Read the model definition and answer for the solid it produces. Units are mm, in the model's axes. Give positions to 0.01 mm unless a question says otherwise; leave off trailing zeros.
```python
from build123d import *

# Parameters (mm, degrees)
SKETCH1_R           = 2
SKETCH1_R_2         = 2.5
SKETCH1_W           = 4
SKETCH1_H           = 7.5
SKETCH1_H_2         = 6
SKETCH1_W_2         = 10
SKETCH1_H_3         = 4
BOSS_EXTRUDE1_DEPTH = 4


with BuildPart() as part:
    # Sketch1 → Boss-Extrude1 (new body)
    with BuildSketch(Plane(origin=(0, 0, 0), x_dir=(1, 0, 0), z_dir=(0, 1, 0))):
        Polygon((-80, -10.54257408), (-80, 9.45742592), (-100, 29.45742592), (-100, 104.45742592), (-80, 124.45742592), (80, 124.45742592), (100, 104.45742592), (100, 29.45742592), (80, 9.45742592), (80, -10.54257408), (100, -30.54257408), (100, -105.54257408), (80, -125.54257408), (-80, -125.54257408), (-100, -105.54257408), (-100, -30.54257408), align=None)
        with Locations(Location((85, 94.45742592, 0), (0, 0, 270))):
            Circle(SKETCH1_R, mode=Mode.SUBTRACT)
        with Locations(Location((85, 46.45742592, 0), (0, 0, 270))):
            Circle(SKETCH1_R, mode=Mode.SUBTRACT)
        with Locations(Location((85, -95.54257408, 0), (0, 0, 90))):
            Circle(SKETCH1_R, mode=Mode.SUBTRACT)
        with Locations(Location((85, -47.54257408, 0), (0, 0, 90))):
            Circle(SKETCH1_R, mode=Mode.SUBTRACT)
        with Locations(Location((-85, 94.45742592, 0), (0, 0, 90))):
            Circle(SKETCH1_R, mode=Mode.SUBTRACT)
        with Locations(Location((-85, 46.45742592, 0), (0, 0, 90))):
            Circle(SKETCH1_R, mode=Mode.SUBTRACT)
        with Locations(Location((-85, -47.54257408, 0), (0, 0, 270))):
            Circle(SKETCH1_R, mode=Mode.SUBTRACT)
        with Locations(Location((-85, -95.54257408, 0), (0, 0, 270))):
            Circle(SKETCH1_R, mode=Mode.SUBTRACT)
        with Locations(Location((60, 114.45742592, 0), (0, 0, 270))):
            Circle(SKETCH1_R_2, mode=Mode.SUBTRACT)
        with Locations(Location((-60, 114.45742592, 0), (0, 0, 90))):
            Circle(SKETCH1_R_2, mode=Mode.SUBTRACT)
        with Locations(Location((-75, -115.54257408, 0), (0, 0, 270))):
            Circle(SKETCH1_R, mode=Mode.SUBTRACT)
        with Locations(Location((-70, -10.54257408, 0), (0, 0, 270))):
            Circle(SKETCH1_R, mode=Mode.SUBTRACT)
        with Locations(Location((75, -115, 0), (0, 0, 270))):
            Circle(SKETCH1_R, mode=Mode.SUBTRACT)
        with Locations(Location((70, -10.54257408, 0), (0, 0, 270))):
            Circle(SKETCH1_R, mode=Mode.SUBTRACT)
        with BuildLine():
            Line((20, -78.04257408), (-20, -78.04257408))
            ThreePointArc((-20, -78.04257408), (-22.5, -75.54257408), (-20, -73.04257408))
            Line((-20, -73.04257408), (20, -73.04257408))
            ThreePointArc((20, -73.04257408), (22.5, -75.54257408), (20, -78.04257408))
        make_face(mode=Mode.SUBTRACT)
        with BuildLine():
            Line((20, 56.95742592), (-20, 56.95742592))
            ThreePointArc((-20, 56.95742592), (-22.5, 54.45742592), (-20, 51.95742592))
            Line((-20, 51.95742592), (20, 51.95742592))
            ThreePointArc((20, 51.95742592), (22.5, 54.45742592), (20, 56.95742592))
        make_face(mode=Mode.SUBTRACT)
        with Locations((95, -41.25)):
            Rectangle(SKETCH1_W, SKETCH1_H, mode=Mode.SUBTRACT)
        with Locations((95, -96.822248533)):
            Rectangle(SKETCH1_W, SKETCH1_H_2, mode=Mode.SUBTRACT)
        with Locations((70, 8)):
            Rectangle(SKETCH1_W_2, SKETCH1_H_3, mode=Mode.SUBTRACT)
        with Locations((95, -56.25)):
            Rectangle(SKETCH1_W, SKETCH1_H, mode=Mode.SUBTRACT)
        with Locations((50, 8)):
            Rectangle(SKETCH1_W_2, SKETCH1_H_3, mode=Mode.SUBTRACT)
        with Locations((95, -84.822248533)):
            Rectangle(SKETCH1_W, SKETCH1_H_2, mode=Mode.SUBTRACT)
        with Locations((-95, -96.822248533)):
            Rectangle(SKETCH1_W, SKETCH1_H_2, mode=Mode.SUBTRACT)
        with Locations((-95, -84.822248533)):
            Rectangle(SKETCH1_W, SKETCH1_H_2, mode=Mode.SUBTRACT)
        with Locations((-95, -56.25)):
            Rectangle(SKETCH1_W, SKETCH1_H, mode=Mode.SUBTRACT)
        with Locations((-95, -41.25)):
            Rectangle(SKETCH1_W, SKETCH1_H, mode=Mode.SUBTRACT)
        with Locations((-50, 8)):
            Rectangle(SKETCH1_W_2, SKETCH1_H_3, mode=Mode.SUBTRACT)
        with Locations((-70, 8)):
            Rectangle(SKETCH1_W_2, SKETCH1_H_3, mode=Mode.SUBTRACT)
    extrude(amount=BOSS_EXTRUDE1_DEPTH)


solid = part.part
```
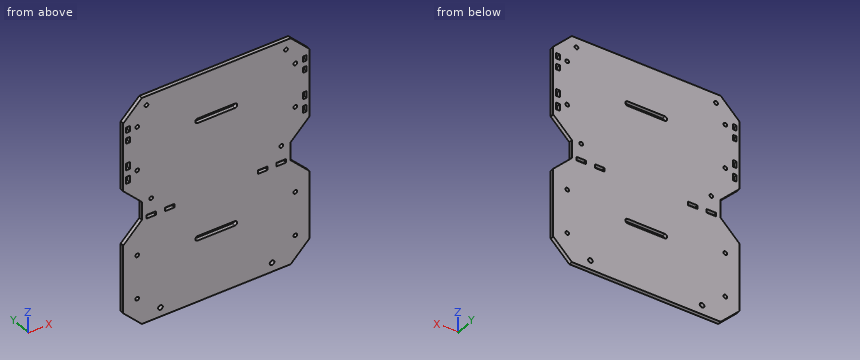
Item 1: Section A-A (y = 1.6) is taken. Give the number of separate pieces and of enclosed holes in the cut face, and give its area (3 significant figures).
Result set:
separate pieces: 1
enclosed holes: 28
area: 46,600 mm2
Item 2: Find the intervals of material crossed by line 1 along Z through (x, y) = (2, 2.85); line 2 along X through (y, z) = (0.6, 57.5); line 3 along Z through (x, y) = (45.5, 2.9), in increasing order.
Result set:
line 1: z = -124.46 to -56.96, -51.96 to 73.04, 78.04 to 125.54
line 2: x = -100 to -97, -93 to 93, 97 to 100
line 3: z = -124.46 to -10, -6 to 125.54
Item 3: Each of these flat-tipped pins is pushed along its axis until it touches: pin 1 Ø4 at (x, z) = (60, -114.46) entering from +Y; pin 2 Ø1.2 at (y, z) = (1.5, -4) entering from -X; pin 3 Ø6 at (x, z) = (-60, -114.46) entering from +Y; pin 4 Ø2 at (x, y) = (94.5, 1) entering from +Z. Where does it stop, or does it pass through?
Result set:
pin 1: passes through
pin 2: stops at x = -80
pin 3: stops at y = 4
pin 4: stops at z = 112.04
